from build123d import *

# Parameters (mm, degrees)
F1_DEPTH = 25


with BuildPart() as f1:
    # F0 (on Top) → F1 (new body)
    with BuildSketch(Plane.XY):
        with BuildLine():
            Line((64.009178, -25.81994), (64.009178, 44.18006))
            ThreePointArc((64.009178, 44.18006), (63.130498, 46.301381), (61.009178, 47.18006))
            Line((61.009178, 47.18006), (51.509178, 47.18006))
            ThreePointArc((51.509178, 47.18006), (50.448518, 46.74072), (50.009178, 45.68006))
            Line((50.009178, 45.68006), (50.009178, 37.18006))
            Line((50.009178, 37.18006), (8.009178, 31.641599))
            Line((8.009178, 31.641599), (8.009178, 25.18006))
            Line((8.009178, 25.18006), (-5.990822, 25.18006))
            Line((-5.990822, 25.18006), (-5.990822, 29.795445))
            Line((-5.990822, 29.795445), (-40.990822, 25.18006))
            Line((-40.990822, 25.18006), (-40.990822, 9.18006))
            Line((-40.990822, 9.18006), (-40.990822, -6.81994))
            Line((-40.990822, -6.81994), (-5.990822, -11.435324))
            Line((-5.990822, -11.435324), (-5.990822, -6.81994))
            Line((-5.990822, -6.81994), (8.009178, -6.81994))
            Line((8.009178, -6.81994), (8.009178, -13.281478))
            Line((8.009178, -13.281478), (50.009178, -18.81994))
            Line((50.009178, -18.81994), (50.009178, -27.31994))
            ThreePointArc((50.009178, -27.31994), (50.448518, -28.3806), (51.509178, -28.81994))
            Line((51.509178, -28.81994), (61.009178, -28.81994))
            ThreePointArc((61.009178, -28.81994), (63.130498, -27.94126), (64.009178, -25.81994))
        make_face()
    extrude(amount=F1_DEPTH)


solid = f1.part
Geometry check sheet. Reference: the model listing, model coordinates, mm. A direction names the side the tool comes from. Round coordinates to 2 decimals unless told otherwise and drop trailing zeros. Order: outer loops, then holes, each group sorted by start corner. A loop starts at its lowest first (then second) coordinate and runs counter-clockwise, first axis right, second up. Notation, with made-up numbers: M 65.25,-40 L 98.25,-40 A6 cw 98.25,-33 Z; hole C 24,25 d1. An arc over 180 degrees is marked long. Write each question's results on one line, items separated by ' | '. Start each with the question number.
1. Set-up check for faces 1 (the face through (1, -6.82, 12)), 2 (the face through (22, 10, 25)), 3 (the face through (1, 25.18, 12)), 4 (the face through (50.009, -23, 12)): record each of +Z, -Z, +X, -X, +Y, -Y from which the full face is reachable in a straight line by a thin tool's end or side.
2. Material ranges on L1, parallel to X at y = -11.5, z = 12.5; L2, parallel to Y at x = 2.5, z = 21.5; L3, parallel to X at y = -25, z = 15.5, recorded low to high. Write a range as from..to.
3. Cross-section at C-C on x = 5. Record the boundary of the cut face in (y, z), plus the area to 3 significant figures.
4. Draft check along X on faces 5 (the face through (56, 47.18, 12)), 6 (the face through (-5.991, -9, 12)), 7 (the face through (50.009, 41, 12)), 8 (the face through (64.009, 9, 12)). Enter one of: pulls with the +X half, pulls with the -X half, needs draft (parallel to the pull), parting line crosses it, or undercut.
5. Go/stop test with flat-tipped pins: P1, Ø5, axis at x = -5.5, z = 9.5, coming from the -Y side; P2, Ø7, axis at x = 3.5, z = 12.5, coming from the +Y side; P3, Ø4, axis at x = -1, z = 11.5, coming from the -Y side. Record where each tip stops, or that it passes through.
6. Cross-section at B-B on y = -20. Record the boundary of the cut face in (x, z).
7. Cross-section at A-A on z = 20.25. Record the boundary of the cut face in (x, y).
Resolved:
1) face 1: +Z, -Z, -Y | face 2: +Z, +X, -X, +Y, -Y | face 3: +Z, -Z, +Y | face 4: +Z, -Z, -X, -Y
2) L1: 8.01..64.01 | L2: -6.82..25.18 | L3: 50.01..64.01
3) outline: M -6.82,0 L 25.18,0 L 25.18,25 L -6.82,25 Z | area: 800 mm2
4) face 5: needs draft | face 6: undercut | face 7: pulls with the -X half | face 8: pulls with the +X half
5) P1: y = -11.44 | P2: y = 25.18 | P3: y = -6.82
6) outline: M 50.01,0 L 64.01,0 L 64.01,25 L 50.01,25 Z
7) outline: M -40.99,-6.82 L -5.99,-11.44 L -5.99,-6.82 L 8.01,-6.82 L 8.01,-13.28 L 50.01,-18.82 L 50.01,-27.32 A1.5 ccw 51.51,-28.82 L 61.01,-28.82 A3 ccw 64.01,-25.82 L 64.01,44.18 A3 ccw 61.01,47.18 L 51.51,47.18 A1.5 ccw 50.01,45.68 L 50.01,37.18 L 8.01,31.64 L 8.01,25.18 L -5.99,25.18 L -5.99,29.8 L -40.99,25.18 Z
